Autodesk Inventor part; units mm, degrees
ref_plane "YZ Plane" through (0, 0, 0) normal (1, 0, 0) x (0, 1, 0)
ref_plane "XZ Plane" through (0, 0, 0) normal (0, 1, 0) x (-1, 0, 0)
ref_plane "XY Plane" through (0, 0, 0) normal (0, 0, 1) x (1, 0, 0)
sketch "Sketch1" plane through (0, 0, 0) normal (0, 1, 0) x (-1, 0, 0)
  line L0 (0, -5.4993) -> (-4.7625, -2.7496)
  line L1 (-4.7625, -2.7496) -> (-4.7625, 2.7496)
  line L2 (-4.7625, 2.7496) -> (0, 5.4993)
  line L3 (0, 5.4993) -> (4.7625, 2.7496)
  line L4 (4.7625, 2.7496) -> (4.7625, -2.7496)
  line L5 (4.7625, -2.7496) -> (0, -5.4993)
  point P0 (0, 0)
  point P1 (0, 0)
  dimension "d0" = 9.525
extrude "Extrusion1" add sketch "Sketch1" along normal blind 20
sketch "Sketch2" plane through (0, 20, 0) normal (0, 1, 0) x (1, 0, 0)
  circle A0 centre (0, 0) radius 4
  dimension "d3" = 8
extrude "Extrusion2" add sketch "Sketch2" along normal blind 5
sketch "Sketch4" plane through (4.7625, 0, 2.7496) normal (0.5, 0, 0.8660254) x (0.8660254, 0, -0.5)
  line L0 (-5.4993, 0) -> (0, 0)
  line L1 (0, 0) -> (0, 20)
  point P0 (-2.7496, 0)
  point P1 (-2.75, 5)
  dimension "d13" = 5
  dimension "d21" = 2.75
hole "Hole1" at (2.3809, 5, 4.1246) direction (-0.5, 0, -0.8660254) diameter 2 end through all countersink diameter 3 countersink angle 82
sketch "Sketch5" plane through (0, 25, 0) normal (0, 1, 0) x (1, 0, 0)
  circle A0 centre (0, 0) radius 4
  circle A1 centre (0, 0) radius 4
extrude "Extrusion4" add sketch "Sketch5" along normal blind 21
sketch "Sketch6" plane through (0, 0, 0) normal (1, 0, 0) x (0, 1, 0)
  line L0 (20, -4) -> (46, -4)
  line L1 (44.414, -4) -> (43.614, -4)
  line L2 (43.614, -4) -> (43.614, -3.5)
  line L3 (43.614, -3.5) -> (44.414, -3.5)
  line L4 (44.414, -3.5) -> (44.414, -4)
  line L5 (46, -4) -> (46, 4)
  line L6 (46, 0) -> (35.8513, 0)
  point P0 (0, 0)
  dimension "d24" = 2.386
  dimension "d25" = 0.8
  dimension "d26" = 7
revolve "Revolution1" cut sketch "Sketch6" angle 360 about axis through (0, 46, 0) along (0, -1, 0)
properties part number "bevel gear shaft connector for versaball" material "Steel"
Check sheet for the modelled part. Datum: model origin and axes. Units: mm. A direction names the side the tool comes from. Round coordinates to 2 decimals unless told otherwise and drop trailing zeros. Order: outer loops, then holes, each group sorted by start corner. A loop starts at its lowest first (then second) coordinate and runs counter-clockwise, first axis right, second up.
Q1. Cross-section at B-B, the plane y = 14. Enter the section's corners in (x, z).
Filled sheet:
outline: (-4.76, -2.75) - (0, -5.5) - (4.76, -2.75) - (4.76, 2.75) - (0, 5.5) - (-4.76, 2.75) - close
Q2. Set-up check for faces 1 (the face through (-0.867, 31.642, -3.905)), 2 (the face through (0, 0, 0)): record each of +Z, -Z, +X, -X, +Y, -Y from which the full face is reachable in a straight line by a thin tool's end or side.
Filled sheet:
face 1: +Y
face 2: +Z, -Z, +X, -X, -Y
Q3. Cross-section at A-A, the plane y = 26. Enter the section's corners in (x, z), plus the area to 3 significant figures.
Filled sheet:
outline: circle Ø8 at (0, 0)
area: 50.3 mm2
Q4. Draft check along Y on faces 3 (the face through (0, 46, 0)), 4 (the face through (-2.348, 9.86, 4.144)), 5 (the face through (1.341, 44.02, -3.233)). Enter one of: pulls with the +Y half, pulls with the -Y half, needs draft (parallel to the pull), parting line crosses it, or undercut.
Filled sheet:
face 3: pulls with the +Y half
face 4: needs draft
face 5: undercut
Q5. Depth check by flat-ended pin: P1, Ø1.5, axis at x = -1, y = 32.5, coming from the +Z side. Enter the tip coordinate at first touch or a pass-through.
Filled sheet:
P1: stops at z = 3.99
Q6. Scan lines: L1, parallel to Y at x = 2.75, z = -2.75; L2, parallel to Y at x = 2.5, z = 2.75; L3, parallel to Z at x = 0, y = 42.5. Record each from-to range of solid material in increasing order.
Filled sheet:
L1: y = 0 to 43.61, 44.41 to 46
L2: y = 0 to 4.39, 5.61 to 43.61, 44.41 to 46
L3: z = -4 to 4
